from build123d import *

# Parameters (mm, degrees)
SKETCH_5_W                      = 10.3
SKETCH_5_H                      = 4.8
EXTRUDE_1_DEPTH                 = 15.75
CUT_EXTRUDE_1_REACH             = 23.278
CUT_EXTRUDE_1_DIRECTION_2_REACH = 23.278
SKETCH_11_R                     = 1.865
CUT_EXTRUDE_2_DEPTH             = 4.8
SKETCH_3_W                      = 0.84
SKETCH_3_H                      = 0.64
SKETCH_4_W                      = 0.84
SKETCH_4_H                      = 0.64
SKETCH_3_3_W                    = 0.84
SKETCH_3_3_H                    = 0.64
EXTRUDE_2_DEPTH                 = 2.5
SKETCH_4_3_W                    = 0.84
SKETCH_4_3_H                    = 0.64
EXTRUDE_3_DEPTH                 = 2.5
SKETCH_12_W                     = 0.84
SKETCH_12_H                     = 0.64
EXTRUDE_4_DEPTH                 = 4
SKETCH_13_R                     = 0.16516852
CUT_EXTRUDE_3_DEPTH             = 1


with BuildPart() as part:
    # Эскиз5 → Вытянуть1 (new body)
    with BuildSketch(Plane(origin=(0, 3.5, 0), x_dir=(-1, 0, 0), z_dir=(0, 1, 0))):
        with Locations((-2.54, -2.4)):
            Rectangle(SKETCH_5_W, SKETCH_5_H)
    extrude(amount=EXTRUDE_1_DEPTH)

    # Вырез-Вытянуть1: up to this face of the body (flat: up to its plane)
    cut_extrude_1_end = Plane(part.part.faces().sort_by_distance((-2.61, 11.375, -2.4))[0])
    # Эскиз10 → Вырез-Вытянуть1 (cut, up to the picked face)
    with BuildSketch(Plane(origin=(0, 0, 0), x_dir=(0, 0, -1), z_dir=(1, 0, 0)), mode=Mode.PRIVATE) as cut_extrude_1_sk1:
        Polygon((0, 19.25), (3.41, 19.25), (3.41, 12.78), (0, 11.5), align=None)
    cut_extrude_1_tool1 = split(extrude(cut_extrude_1_sk1.sketch, amount=-CUT_EXTRUDE_1_REACH, mode=Mode.PRIVATE), bisect_by=cut_extrude_1_end, keep=Keep.BOTH, mode=Mode.PRIVATE)
    add(cut_extrude_1_tool1.solids().sort_by(Axis((0, 15.685398, -1.653842), (-1, 0, 0)))[0], mode=Mode.SUBTRACT)

    # Вырез-Вытянуть1 direction 2: up to this face of the body (flat: up to its plane)
    cut_extrude_1_direction_2_end = Plane(part.part.faces().sort_by_distance((7.69, 11.375, -2.4))[0])
    # Эскиз10 → Вырез-Вытянуть1 direction 2 (cut, up to the picked face)
    with BuildSketch(Plane(origin=(0, 0, 0), x_dir=(0, 0, -1), z_dir=(1, 0, 0)), mode=Mode.PRIVATE) as cut_extrude_1_direction_2_sk1:
        Polygon((0, 19.25), (3.41, 19.25), (3.41, 12.78), (0, 11.5), align=None)
    cut_extrude_1_direction_2_tool1 = split(extrude(cut_extrude_1_direction_2_sk1.sketch, amount=CUT_EXTRUDE_1_DIRECTION_2_REACH, mode=Mode.PRIVATE), bisect_by=cut_extrude_1_direction_2_end, keep=Keep.BOTH, mode=Mode.PRIVATE)
    add(cut_extrude_1_direction_2_tool1.solids().sort_by(Axis((0, 15.685398, -1.653842), (1, 0, 0)))[0], mode=Mode.SUBTRACT)

    # Эскиз11 → Вырез-Вытянуть2 (cut)
    with BuildSketch(Plane.XY):
        with Locations((2.54, 15.77)):
            Circle(SKETCH_11_R)
    extrude(amount=-CUT_EXTRUDE_2_DEPTH, mode=Mode.SUBTRACT)

    # По траектории1: sweep along a path in Эскиз8
    with BuildLine(Plane(origin=(0, 0, 0), x_dir=(0, 0, -1), z_dir=(1, 0, 0))) as sweep_1_path:
        Line((0, 0), (0.6, 0))
        ThreePointArc((0.6, 0), (1.307106781, 0.292893219), (1.6, 1))
        Line((1.6, 1), (1.6, 3.5))
    # Эскиз3 → По траектории1 (sweep)
    with BuildSketch(Plane.XY):
        Rectangle(SKETCH_3_W, SKETCH_3_H)
        with Locations((5.08, 0)):
            Rectangle(SKETCH_3_W, SKETCH_3_H)
    sweep(path=sweep_1_path.line)

    # По траектории2: sweep along a path in Эскиз9
    with BuildLine(Plane(origin=(0, 0, 0), x_dir=(0, 0, -1), z_dir=(1, 0, 0))) as sweep_2_path:
        Line((0, -2.54), (0.6, -2.54))
        ThreePointArc((0.6, -2.54), (1.307106781, -2.247106781), (1.6, -1.54))
        Line((1.6, -1.54), (1.6, 4.77))
    # Эскиз4 → По траектории2 (sweep)
    with BuildSketch(Plane.XY):
        with Locations((2.54, -2.54)):
            Rectangle(SKETCH_4_W, SKETCH_4_H)
    sweep(path=sweep_2_path.line)

    # Эскиз3<3> → Вытянуть2 (add)
    with BuildSketch(Plane.XY):
        Rectangle(SKETCH_3_3_W, SKETCH_3_3_H)
        with Locations((5.08, 0)):
            Rectangle(SKETCH_3_3_W, SKETCH_3_3_H)
    extrude(amount=EXTRUDE_2_DEPTH)

    # Эскиз4<3> → Вытянуть3 (add)
    with BuildSketch(Plane.XY):
        with Locations((2.54, -2.54)):
            Rectangle(SKETCH_4_3_W, SKETCH_4_3_H)
    extrude(amount=EXTRUDE_3_DEPTH)

    # Эскиз12 → Вытянуть4 (add)
    with BuildSketch(Plane.XY.offset(2.5)):
        Rectangle(SKETCH_12_W, SKETCH_12_H)
        with Locations((5.08, 0)):
            Rectangle(SKETCH_12_W, SKETCH_12_H)
        with Locations((2.54, -2.54)):
            Rectangle(SKETCH_12_W, SKETCH_12_H)
    extrude(amount=EXTRUDE_4_DEPTH)

    # Эскиз13 → Вырез-Вытянуть3 (cut)
    with BuildSketch(Plane.XY.offset(6.5)):
        Circle(SKETCH_13_R)
    extrude(amount=-CUT_EXTRUDE_3_DEPTH, mode=Mode.SUBTRACT)


solid = part.part
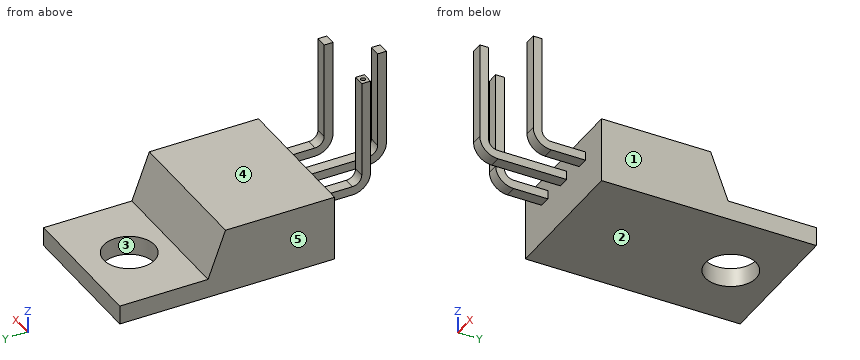
Work out the finished part from the listing and answer in its coordinate system (mm). Face numbers are marked on the shaded views. A direction names the side the tool comes from. Round coordinates to 2 decimals unless told otherwise and drop trailing zeros. Order: outer loops, then holes, each group sorted by start corner. A loop starts at its lowest first (then second) coordinate and runs counter-clockwise, first axis right, second up. Notation, with made-up numbers: M -4,-29 L 33,-29 A20 ccw 33,-11 Z; hole C -8.5,56 d11. An arc over 180 degrees is marked long. Put each result on its own line as item: value. Start each with the question number.
Q1. Section A-A, the plane x = 2.54 is taken. Write down the section's boundary in (y, z) (3 decimals), and give its area (3 significant figures).
Q2. Section B-B, the plane y = 1.25 is taken. Write down the section's boundary in (x, z).
Q3. Section D-D, the plane y = 15.77 is taken. Write down the section's boundary in (x, z) (3 decimals).
Q4. For a pull along X with two mould halves and no side action, classify the marked faces 1, 2 and 3 as pulls with the +X half, pulls with the -X half, needs draft (parallel to the pull), parting line crosses it, or undercut.
Q5. Flat-ended cylindrical pins translate along their axes: pin 1 (3 mm diameter, centred on y = 0, z = 4.5, fed in from +X); pin 2 (5 mm diameter, centred on y = 0.5, z = 2, fed in from -X); pin 3 (4 mm diameter, centred on x = 1.5, y = 6.5, fed in from +Z). Find the tip coordinate at first contact, or state that the pin passes through.
Q6. A tool of negligible diameter and unlimited length cuts with its end or side. For the marked faces 4 and 5, from which of +Z, -Z, +X, -X, +Y, -Y can it reach the whole face along a straight path? Write none if from no direction.
Q7. Section C-C, the plane z = 0.75 is taken. Write down the section's boundary in (x, y), and give its area (3 significant figures).
Q8. Straight lines are drawn through the part: L1, parallel to Y at x = 2.54, z = -4.35 (3 decimals); L2, parallel to Y at x = 0, z = 6.05; L3, parallel to Z at x = 7.25, y = 5. For each, find the intervals that lie inside material, in ascending order. Write a range as [from, to].
Findings below:
1. outline: M -2.86,-0.6 A1.32 ccw -1.54,-1.92 L 3.5,-1.92 L 3.5,-4.8 L 13.905,-4.8 L 13.905,-3.41 L 12.78,-3.41 L 11.5,0 L 3.5,0 L 3.5,-1.28 L -1.54,-1.28 A0.68 cw -2.22,-0.6 L -2.22,6.5 L -2.86,6.5 Z; M 17.635,-4.8 L 19.25,-4.8 L 19.25,-3.41 L 17.635,-3.41 Z
1. area: 54.9 mm^2
2. outline: M -0.42,-1.92 L 0.42,-1.92 L 0.42,-1.28 L -0.42,-1.28 Z; M 2.12,-1.92 L 2.96,-1.92 L 2.96,-1.28 L 2.12,-1.28 Z; M 4.66,-1.92 L 5.5,-1.92 L 5.5,-1.28 L 4.66,-1.28 Z
3. outline: M -2.61,-4.8 L 0.675,-4.8 L 0.675,-3.41 L -2.61,-3.41 Z; M 4.405,-4.8 L 7.69,-4.8 L 7.69,-3.41 L 4.405,-3.41 Z
4. face 1: pulls with the +X half
4. face 2: needs draft
4. face 3: undercut
5. pin 1: stops at x = 5.5
5. pin 2: stops at x = -0.42
5. pin 3: stops at z = 0
6. face 4: +Z, +X, -X, +Y
6. face 5: +Z, -Z, -X, +Y, -Y
7. outline: M -0.42,-0.32 L 0.42,-0.32 L 0.42,0.32 L -0.42,0.32 Z; M 2.12,-2.86 L 2.96,-2.86 L 2.96,-2.22 L 2.12,-2.22 Z; M 4.66,-0.32 L 5.5,-0.32 L 5.5,0.32 L 4.66,0.32 Z
7. area: 1.61 mm^2
8. L1: y = [3.5, 13.905], [17.635, 19.25]
8. L2: y = [-0.32, -0.17], [0.17, 0.32]
8. L3: z = [-4.8, 0]
